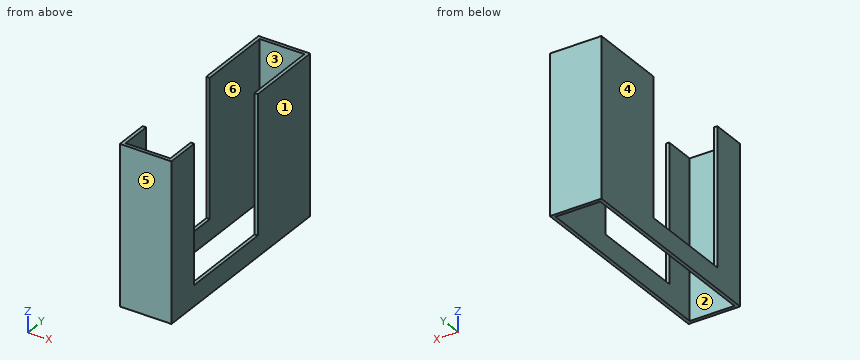
from build123d import *

# Parameters (mm, degrees)
SKETCH1_W           = 75
SKETCH1_H           = 305
SKETCH1_W_2         = 65
SKETCH1_H_2         = 295
BOSS_EXTRUDE1_DEPTH = 230
SKETCH2_W           = 200
SKETCH2_H           = 140
CUT_EXTRUDE1_DEPTH  = 286.974212124


with BuildPart() as part:
    # Sketch1 → Boss-Extrude1 (new body)
    with BuildSketch(Plane.XY):
        Rectangle(SKETCH1_W, SKETCH1_H)
        Rectangle(SKETCH1_W_2, SKETCH1_H_2, mode=Mode.SUBTRACT)
    extrude(amount=BOSS_EXTRUDE1_DEPTH)

    # Sketch2 → Cut-Extrude1 (cut, through all)
    with BuildSketch(Plane(origin=(37.5, 0, 0), x_dir=(0, 0, -1), z_dir=(1, 0, 0))):
        with Locations((-130, -32.5)):
            Rectangle(SKETCH2_W, SKETCH2_H)
    extrude(amount=-CUT_EXTRUDE1_DEPTH, mode=Mode.SUBTRACT)


solid = part.part
Work out the finished part from the listing and answer in its coordinate system (mm). Face numbers are marked on the shaded views. A direction names the side the tool comes from. Give positions to 0.01 mm unless a question says otherwise; leave off trailing zeros. Write each loop counter-clockwise with the first axis right and the second up, starting at its lowest first coordinate (ties: lowest second). Pieces come first, ordered by that corner, then holes.
Q1. Straight lines are drawn through the part: L1, parallel to X at y = 76, z = 154.5; L2, parallel to Y at x = 6.5, z = 156; L3, parallel to Z at x = 33.5, y = -85. For each, find the intervals that lie inside material, in ascending order.
Answer:
L1: x = -37.5 to -32.5, 32.5 to 37.5
L2: y = -152.5 to -147.5, 147.5 to 152.5
L3: z = 0 to 30
Q2. The part is cut by section B-B on y = -132. Give the vertices of the cut face in (x, z), and give its area (3 significant figures).
Answer:
outline: (-37.5, 0) - (-32.5, 0) - (-32.5, 230) - (-37.5, 230) - close; (32.5, 0) - (37.5, 0) - (37.5, 230) - (32.5, 230) - close
area: 2,300 mm2
Q3. For a pull along Y with two mould halves and no side action, classify the marked faces 3, 4, 5 and 6 as released by +Y, released by -Y, zero draft, split by the parting line, or undercut.
Answer:
face 3: undercut
face 4: zero draft
face 5: released by -Y
face 6: undercut
Q4. A tool of negligible diameter and unlimited length cuts with its end or side. For the marked faces 1 and 2, from which of +Z, -Z, +X, -X, +Y, -Y can it reach the whole face along a straight path? Write none if from no direction.
Answer:
face 1: +Z, -Z, +X, +Y, -Y
face 2: +Z, -Z
Q5. Given pin 1 (2.5 mm diameter, centred on x = -36, y = -49, fed in from +Z); pin 2 (3 mm diameter, centred on x = -30, y = 3.5, fed in from +Z), each flat-ended and moving along its own axis, determine where each tip first touches the part or whether it passes through.
Answer:
pin 1: stops at z = 30
pin 2: passes through
Q6. The part is cut by section A-A on x = -24. Give the vertices of the cut face in (y, z), and give its area (3 significant figures).
Answer:
outline: (-152.5, 0) - (-147.5, 0) - (-147.5, 230) - (-152.5, 230) - close; (147.5, 0) - (152.5, 0) - (152.5, 230) - (147.5, 230) - close
area: 2,300 mm2
Q7. The part is cut by section C-C on z = 176. Give the vertices of the cut face in (x, y).
Answer:
outline: (-37.5, -152.5) - (37.5, -152.5) - (37.5, -102.5) - (32.5, -102.5) - (32.5, -147.5) - (-32.5, -147.5) - (-32.5, -102.5) - (-37.5, -102.5) - close; (-37.5, 37.5) - (-32.5, 37.5) - (-32.5, 147.5) - (32.5, 147.5) - (32.5, 37.5) - (37.5, 37.5) - (37.5, 152.5) - (-37.5, 152.5) - close
